Read the model definition and answer for the solid it produces. Units are mm, in the model's axes. A direction names the side the tool comes from. Coordinates: 2 decimals unless noted, no trailing zeros. Write each loop counter-clockwise with the first axis right and the second up, starting at its lowest first coordinate (ties: lowest second). Pieces come first, ordered by that corner, then holes.
(1) The part is cut by section C-C, the plane y = 19. Determine the outline of the cut face in (x, z), and give its area (3 significant figures).
(2) Determine the mould class of faces 1 (the flat face through (-71.205, -19.788, 29.499)), 2 (the flat face through (-83.078, -46.018, 32.935)), 3 (the flat face through (-85, -53.74, 38)), 4 (the flat face through (-9, -9, 76.2)) for opening direction Z: pulls with the +Z half, pulls with the -Z half, needs draft (parallel to the pull), parting line crosses it, or undercut.
(3) Given pin 1 (6 mm diameter, centred on y = -50, z = 25.5, fed in from +X); pin 2 (5 mm diameter, centred on y = -33.5, z = 29, fed in from -X); pin 3 (8 mm diameter, centred on x = -20, z = 38, fed in from -Y), each flat-ended and moving along its own axis, determine where each tip first touches the part or whether it passes through.
(4) The part is cut by section A-A, the plane x = 0. Determine the outline of the cut face in (y, z).
(5) The part is cut by section B-B, the plane z = 24. Determine the outline of the cut face in (x, y), and give its area (3 significant figures).
(6) The part is cut by section D-D, the plane z = 61. Determine the outline of the cut face in (x, y).
(7) Which of the six approach directions +Z, -Z, +X, -X, +Y, -Y give full straight-line access (tool end or side, diameter ignored) to faces 5 (the flat face through (20, -42.178, 46)), 6 (the flat face through (-90, -38.078, 38)), 7 (the flat face through (-71.72, -19.79, 38.04))?
(8) Straight lines are drawn through the part: line 1 along X through (y, z) = (-15, 23); line 2 along X through (y, z) = (-8.5, 60.5); line 3 along Z through (x, y) = (0, -14). For each, find the intervals that lie inside material, in ascending order.
```python
from build123d import *

# Parameters (mm, degrees)
F0_R     = 8.190345508
F0_R_2   = 18.0615768445
F0_W     = 25.6181135774
F0_H     = 4.1002519429
F1_DEPTH = 76.2
F3_DEPTH = 88.9068820903
F4_R     = 22.0566851371
F5_DEPTH = 88.9068820903


with BuildPart() as f1:
    # F0 (on Top) → F1 (new body)
    with BuildSketch(Plane.XY):
        Polygon((91.2738516927, 35.1657494903), (-74.9807953835, 35.1657494903), (-74.9807953835, -38.0775630474), (-49.3626818061, -38.0775630474), (-49.3626818061, -42.1778149903), (91.2738516927, -42.1778149903), align=None)
        with Locations((-34.8990187049, -4.2046573944)):
            Circle(F0_R, mode=Mode.SUBTRACT)
        with Locations((45.6959344447, -4.3521164916)):
            Circle(F0_R_2, mode=Mode.SUBTRACT)
        Polygon((-74.9807953835, -42.1778149903), (-74.9807953835, -38.0775630474), (-106.267772615, -38.0775630474), (-106.267772615, -53.7401326001), (-49.3626818061, -53.7401326001), (-49.3626818061, -42.1778149903), align=None)
        with Locations((-62.1717385948, -40.1276890188)):
            Rectangle(F0_W, F0_H)
    extrude(amount=F1_DEPTH)

    # F2 (on face) → F3 (cut, through all)
    with BuildSketch(Plane.XZ.offset(53.7401326001)):
        Polygon((-64.0935031806, 34.5261069518), (-84.0708138313, 43.7335528065), (-82.05604052, 21.8289713563), align=None)
    extrude(amount=-F3_DEPTH, mode=Mode.SUBTRACT)

    # F4 (on face) → F5 (cut, through all)
    with BuildSketch(Plane(origin=(0, 35.1657494903, 0), x_dir=(-1, 0, 0), z_dir=(0, 1, 0))):
        with Locations((0, 28.9242751896)):
            Circle(F4_R)
    extrude(amount=-F5_DEPTH, mode=Mode.SUBTRACT)


solid = f1.part
```
Computed:
1. outline: (-74.98, 0) - (91.27, 0) - (91.27, 76.2) - (-74.98, 76.2) - (-74.98, 39.54) - (-64.09, 34.53) - (-74.98, 26.83) - close; hole circle Ø44.11 at (0, 28.92)
1. area: 11,100 mm2
2. face 1: undercut
2. face 2: undercut
2. face 3: needs draft
2. face 4: pulls with the +Z half
3. pin 1: stops at x = -49.36
3. pin 2: stops at x = -74.98
3. pin 3: stops at y = -42.18
4. outline: (-42.18, 0) - (35.17, 0) - (35.17, 6.87) - (-42.18, 6.87) - close; (-42.18, 50.98) - (35.17, 50.98) - (35.17, 76.2) - (-42.18, 76.2) - close
5. outline: (-106.27, -53.74) - (-82.26, -53.74) - (-82.26, -38.08) - (-106.27, -38.08) - close; (-78.98, -53.74) - (-49.36, -53.74) - (-49.36, -42.18) - (-21.5, -42.18) - (-21.5, 35.17) - (-74.98, 35.17) - (-74.98, -38.08) - (-78.98, -38.08) - close; (21.5, -42.18) - (91.27, -42.18) - (91.27, 35.17) - (21.5, 35.17) - close; hole circle Ø16.38 at (-34.9, -4.2); hole circle Ø36.12 at (45.7, -4.35)
5. area: 9,030 mm2
6. outline: (-106.27, -53.74) - (-49.36, -53.74) - (-49.36, -42.18) - (91.27, -42.18) - (91.27, 35.17) - (-74.98, 35.17) - (-74.98, -38.08) - (-106.27, -38.08) - close; hole circle Ø16.38 at (-34.9, -4.2); hole circle Ø36.12 at (45.7, -4.35)
7. face 5: +Z, -Z, +X, -Y
7. face 6: +Z, -Z, -X, +Y
7. face 7: +Y, -Y
8. line 1: x = -74.98 to -21.25, 21.25 to 31.11, 60.29 to 91.27
8. line 2: x = -74.98 to -41.87, -27.93 to 28.12, 63.27 to 91.27
8. line 3: z = 0 to 6.87, 50.98 to 76.2
